Input: part model. Units: mm. Frame: model coordinates. Face numbers are marked on the shaded views. A direction names the side the tool comes from. Give positions to 0.01 mm unless a question says otherwise; leave off trailing zeros. Loops run counter-clockwise (first coordinate to the right, second up) from the corner with the lowest first, then second, coordinate; pieces in that order, holes last. Notation, with made-up numbers: (-17, 54) -> (3, 54) arc R23 ccw to (3, 88) -> close; hole circle Ø4 at (59.25, 49). An arc over 180 degrees is marked (long way). Answer as a JSON object with one key per item and string values.
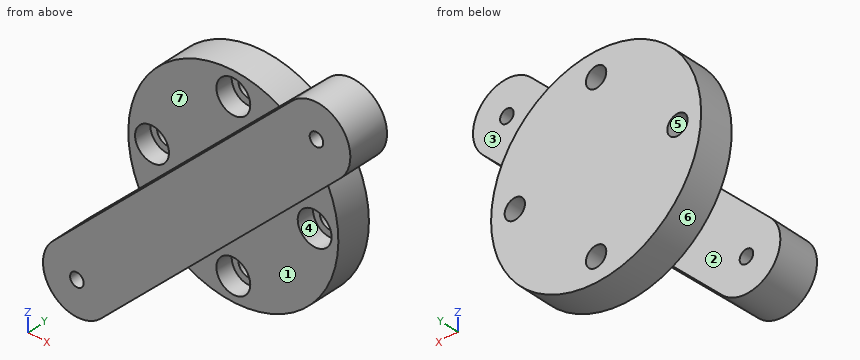
```python
from build123d import *

# Parameters (mm, degrees)
SKETCH1_R           = 31
BOSS_EXTRUDE1_DEPTH = 10
SKETCH2_R           = 3
CUT_EXTRUDE11_DEPTH = 10
SKETCH5_R           = 5
CUT_EXTRUDE14_DEPTH = 5
SKETCH6_R           = 2
BOSS_EXTRUDE5_DEPTH = 12


with BuildPart() as part:
    # Sketch1 → Boss-Extrude1 (new body)
    with BuildSketch(Plane(origin=(0, 0, 0), x_dir=(1, 0, 0), z_dir=(0, 1, 0))):
        with Locations(Location((0, 0, 0), (0, 0, 270))):
            Circle(SKETCH1_R)
    extrude(amount=BOSS_EXTRUDE1_DEPTH)

    # Sketch2 → Cut-Extrude11 (cut)
    with BuildSketch(Plane(origin=(0, 10, 0), x_dir=(1, 0, 0), z_dir=(0, 1, 0))):
        with Locations(Location((0, 24, 0), (0, 0, 270))):
            Circle(SKETCH2_R)
        with Locations(Location((24, 0, 0), (0, 0, 270))):
            Circle(SKETCH2_R)
        with Locations(Location((0, -24, 0), (0, 0, 270))):
            Circle(SKETCH2_R)
        with Locations(Location((-24, 0, 0), (0, 0, 270))):
            Circle(SKETCH2_R)
    extrude(amount=-CUT_EXTRUDE11_DEPTH, mode=Mode.SUBTRACT)

    # Sketch5 → Cut-Extrude14 (cut)
    with BuildSketch(Plane(origin=(0, 0, 0), x_dir=(1, 0, 0), z_dir=(0, 1, 0))):
        with Locations(Location((0, 24, 0), (0, 0, 270))):
            Circle(SKETCH5_R)
        with Locations(Location((24, 0, 0), (0, 0, 270))):
            Circle(SKETCH5_R)
        with Locations(Location((0, -24, 0), (0, 0, 270))):
            Circle(SKETCH5_R)
        with Locations(Location((-24, 0, 0), (0, 0, 270))):
            Circle(SKETCH5_R)
    extrude(amount=CUT_EXTRUDE14_DEPTH, mode=Mode.SUBTRACT)

    # Sketch6 → Boss-Extrude5 (add)
    with BuildSketch(Plane(origin=(0, 0, 0), x_dir=(1, 0, 0), z_dir=(0, 1, 0))):
        with BuildLine():
            Line((28.284271247, -42.426406871), (-42.426406871, 28.284271247))
            ThreePointArc((-42.426406871, 28.284271247), (-42.426406871, 42.426406871), (-28.284271247, 42.426406871))
            Line((-28.284271247, 42.426406871), (42.426406871, -28.284271247))
            ThreePointArc((42.426406871, -28.284271247), (42.426406871, -42.426406871), (28.284271247, -42.426406871))
        make_face()
        with Locations(Location((-35.355339059, 35.355339059, 0), (0, 0, 270))):
            Circle(SKETCH6_R, mode=Mode.SUBTRACT)
        with Locations(Location((35.355339059, -35.355339059, 0), (0, 0, 270))):
            Circle(SKETCH6_R, mode=Mode.SUBTRACT)
    extrude(amount=-BOSS_EXTRUDE5_DEPTH)


solid = part.part
```
Q1. Section D-D, the plane x = 9. Return the cut outline in (y, z), then the cut area to 3 significant figures.
Evaluation:
{"outline": "(-12, -5.14) -> (0, -5.14) -> (0, -29.66) -> (10, -29.66) -> (10, 29.66) -> (0, 29.66) -> (0, 23.14) -> (-12, 23.14) -> close", "area": "933 mm2"}
Q2. Pin query (flat end, axial travel): pin 1 (22.5 mm diameter, centred on x = 8.5, z = -9, fed in from -Y); pin 2 (11 mm diameter, centred on x = 22, z = 0, fed in from -Y); pin 3 (5.5 mm diameter, centred on x = 24, z = 0, fed in from -Y); pin 4 (10 mm diameter, centred on x = 14.5, y = -9.5, fed in from +Z). Return the tip coordinate at first contact, or that it passes through.
Evaluation:
{"pin 1": "stops at y = -12", "pin 2": "stops at y = 0", "pin 3": "passes through", "pin 4": "stops at z = 33.64"}
Q3. Section A-A, the plane x = -25.5. Return the cut outline in (y, z), then the cut area to 3 significant figures.
Evaluation:
{"outline": "(-12, -39.64) -> (0, -39.64) -> (0, -17.63) -> (10, -17.63) -> (10, -2.6) -> (5, -2.6) -> (5, -4.77) -> (0, -4.77) -> (0, -11.36) -> (-12, -11.36) -> close; (0, 4.77) -> (5, 4.77) -> (5, 2.6) -> (10, 2.6) -> (10, 17.63) -> (0, 17.63) -> close", "area": "618 mm2"}
Q4. Section B-B, the plane z = 24. Return the cut outline in (x, y), then the cut area to 3 significant figures.
Evaluation:
{"outline": "(-19.62, 0) -> (-5, 0) -> (-5, 5) -> (-3, 5) -> (-3, 10) -> (-19.62, 10) -> close; (3, 5) -> (5, 5) -> (5, 0) -> (9.86, 0) -> (9.86, -12) -> (38.14, -12) -> (38.14, 0) -> (19.62, 0) -> (19.62, 10) -> (3, 10) -> close", "area": "652 mm2"}
Q5. Draft query along X for the marked faces 5, 6 and 7. Return one class per face: +X half, -X half, draft (parallel to the pull), parting line (faces both ways), or undercut.
Evaluation:
{"face 5": "undercut", "face 6": "parting line", "face 7": "draft"}
Q6. Section C-C, the plane z = 0. Return the cut outline in (x, y), then the cut area to 3 significant figures.
Evaluation:
{"outline": "(-31, 0) -> (-29, 0) -> (-29, 5) -> (-27, 5) -> (-27, 10) -> (-31, 10) -> close; (-21, 5) -> (-19, 5) -> (-19, 0) -> (-14.14, 0) -> (-14.14, -12) -> (14.14, -12) -> (14.14, 0) -> (19, 0) -> (19, 5) -> (21, 5) -> (21, 10) -> (-21, 10) -> close; (27, 5) -> (29, 5) -> (29, 0) -> (31, 0) -> (31, 10) -> (27, 10) -> close", "area": "799 mm2"}
Q7. Ray query, line 1 along X through (y, z) = (3.25, 0); line 2 along X through (y, z) = (7.6, 0); line 3 along Y through (x, z) = (-23, -34.5). Return the intervals inside material, ascending.
Evaluation:
{"line 1": "x = -31 to -29, -19 to 19, 29 to 31", "line 2": "x = -31 to -27, -21 to 21, 27 to 31", "line 3": "y = -12 to 0"}
Q8. Access query for the marked faces 1, 2, 3 and 4. Directions: +Z, -Z, +X, -X, +Y, -Y. A direction counts if a zero-diameter tool reaches every point of the face in a straight line with its end or side. Return the directions, or none.
Evaluation:
{"face 1": "-Z, +X, -Y", "face 2": "-Z, -X, +Y", "face 3": "+Z, +X, +Y", "face 4": "-Y"}
